```python
from build123d import *

# Parameters (mm, degrees)
BASPROSKE_W             = 5
BASPROSKE_H             = 10.125
TOOTHCUT_DEPTH          = 16.166781135
TEETHCUTS_COUNT         = 13
TEETHCUTS_ANGLE         = 270
BORSKE_R                = 2.5
BORE_DEPTH              = 50.0000508
ENL_V_START             = -10
ENL_V_MAT_EXTRU_1_DEPTH = 10
ESQUISSE2_R             = 1.5
BOSS_EXTRU_1_DEPTH      = 5
BOSS_EXTRU_2_START      = -1
ESQUISSE3_R             = 2.5
BOSS_EXTRU_2_DEPTH      = 4
ESQUISSE4_R             = 1
ENL_V_MAT_EXTRU_2_DEPTH = 10
CONG_1_R                = 5
CONG_2_R                = 8
ENL_V_MAT_EXTRU_4_DEPTH = 2.1
ESQUISSE8_R             = 0.515
ENL_V_MAT_EXTRU_5_DEPTH = 33.049570744


with BuildPart() as part:
    # BasProSke → Base-Revolve (revolve)
    with BuildSketch(Plane(origin=(0, 0, 0), x_dir=(1, 0, 0), z_dir=(0, 1, 0)), mode=Mode.PRIVATE) as base_revolve_sk:
        with Locations((2.5, 5.0625)):
            Rectangle(BASPROSKE_W, BASPROSKE_H)
    revolve(base_revolve_sk.sketch.rotate(Axis((-10, 0, 0), (1, 0, 0)), 180), axis=Axis((-10, 0, 0), (1, 0, 0)))

    # TooCutSke → ToothCut (cut, through all)
    with BuildSketch(Plane(origin=(0, 0, 0), x_dir=(0, 0, -1), z_dir=(1, 0, 0))):
        with BuildLine():
            ThreePointArc((0.588166249, 7.56993481), (0, 7.59275), (-0.588166249, 7.56993481))
            ThreePointArc((-0.588166249, 7.56993481), (-0.930156891, 8.896709021), (-1.743114395, 9.999608611))
            ThreePointArc((-1.743114395, 9.999608611), (0, 10.1504), (1.743114395, 9.999608611))
            ThreePointArc((1.743114395, 9.999608611), (0.930156891, 8.896709021), (0.588166249, 7.56993481))
        make_face()
    toothcut = extrude(amount=TOOTHCUT_DEPTH, mode=Mode.SUBTRACT)

    # TeethCuts: ToothCut ×13 about axis
    teethcuts_axis = Axis((-10, 0, 0), (1, 0, 0))
    for i in range(1, TEETHCUTS_COUNT):
        add(toothcut.rotate(teethcuts_axis, i * TEETHCUTS_ANGLE / (TEETHCUTS_COUNT - 1)), mode=Mode.SUBTRACT)

    # BorSke → Bore (cut, symmetric)
    with BuildSketch(Plane(origin=(0, 0, 0), x_dir=(0, 0, -1), z_dir=(1, 0, 0))):
        with Locations(Location((0, 0, 0), (0, 0, 180))):
            Circle(BORSKE_R)
    extrude(amount=BORE_DEPTH, both=True, mode=Mode.SUBTRACT)

    # Esquisse1 → Enlèv. mat.-Extru.1 (cut)
    with BuildSketch(Plane(origin=(5, 0, 0), x_dir=(0, 0, -1), z_dir=(1, 0, 0)).offset(ENL_V_START)):
        with BuildLine():
            ThreePointArc((7.56993481, 0.588166249), (5.368885013, 5.368885013), (0.588166249, 7.56993481))
            ThreePointArc((0.588166249, 7.56993481), (0.923336805, 8.882279141), (1.719727125, 9.977883724))
            ThreePointArc((1.719727125, 9.977883724), (7.15945616, 7.15945616), (9.977883724, 1.719727125))
            ThreePointArc((9.977883724, 1.719727125), (8.882279141, 0.923336805), (7.56993481, 0.588166249))
        make_face()
    extrude(amount=ENL_V_MAT_EXTRU_1_DEPTH, mode=Mode.SUBTRACT)

    # Esquisse2 → Boss.-Extru.1 (add, through all)
    with BuildSketch(Plane(origin=(5, 0, 0), x_dir=(0, 0, -1), z_dir=(1, 0, 0))):
        with BuildLine():
            Line((16.142135624, 21.46674159), (2, 7.324605966))
            ThreePointArc((2, 7.324605966), (5.368885013, 5.368885013), (7.324605966, 2))
            Line((7.324605966, 2), (21.46674159, 16.142135624))
            ThreePointArc((21.46674159, 16.142135624), (21.46674159, 21.46674159), (16.142135624, 21.46674159))
        make_face()
        with Locations((18.804438607, 18.804438607)):
            Circle(ESQUISSE2_R, mode=Mode.SUBTRACT)
    extrude(amount=-BOSS_EXTRU_1_DEPTH)

    # Esquisse3 → Boss.-Extru.2 (add, through all)
    with BuildSketch(Plane(origin=(5, 0, 0), x_dir=(0, 0, -1), z_dir=(1, 0, 0)).offset(BOSS_EXTRU_2_START)):
        with Locations(Location((0, 0, 0), (0, 0, 180))):
            Circle(ESQUISSE3_R)
    extrude(amount=-BOSS_EXTRU_2_DEPTH)

    # Esquisse4 → Enlèv. mat.-Extru.2 (cut)
    with BuildSketch(Plane(origin=(4, 0, 0), x_dir=(0, 0, -1), z_dir=(1, 0, 0))):
        Circle(ESQUISSE4_R)
    extrude(amount=-ENL_V_MAT_EXTRU_2_DEPTH, mode=Mode.SUBTRACT)

    # Congé1
    cong_1_edges = [part.edges().sort_by_distance(p)[0] for p in [
        (2.5, 7.324605966, -2),
    ]]
    fillet(cong_1_edges, radius=CONG_1_R)

    # Congé2
    cong_2_edges = [part.edges().sort_by_distance(p)[0] for p in [
        (2.5, 2, -7.324605966),
    ]]
    fillet(cong_2_edges, radius=CONG_2_R)

    # Esquisse6 → Enlèv. mat.-Extru.4 (cut)
    with BuildSketch(Plane(origin=(5, 0, 0), x_dir=(0, 0, -1), z_dir=(1, 0, 0))):
        with BuildLine():
            Line((-0.486746212, 3.465988766), (1.140136775, 5.092871753))
            ThreePointArc((1.140136775, 5.092871753), (4.507727263, 5.08472958), (4.91940393, 1.742386942))
            Line((4.91940393, 1.742386942), (3.499344691, -0.067725445))
            ThreePointArc((3.499344691, -0.067725445), (2.619022446, -2.321792719), (0.486746212, -3.465988766))
            Line((0.486746212, -3.465988766), (-1.140072016, -5.092806994))
            ThreePointArc((-1.140072016, -5.092806994), (-4.507662796, -5.08478673), (-4.919460458, -1.742458998))
            Line((-4.919460458, -1.742458998), (-3.499344691, 0.067725445))
            ThreePointArc((-3.499344691, 0.067725445), (-2.619022446, 2.321792719), (-0.486746212, 3.465988766))
        make_face()
    extrude(amount=-ENL_V_MAT_EXTRU_4_DEPTH, mode=Mode.SUBTRACT)

    # Esquisse8 → Enlèv. mat.-Extru.5 (cut, through all)
    with BuildSketch(Plane(origin=(2.9, 0, 0), x_dir=(0, 0, -1), z_dir=(1, 0, 0))):
        with Locations((-2.81931973, -3.180241541)):
            Circle(ESQUISSE8_R)
        with Locations((2.81931973, 3.180241541)):
            Circle(ESQUISSE8_R)
    extrude(amount=-ENL_V_MAT_EXTRU_5_DEPTH, mode=Mode.SUBTRACT)


solid = part.part
```
Model file for the job. Use its own axes, mm. A direction names the side the tool comes from. Coordinates: 2 decimals unless noted, no trailing zeros. Write each loop counter-clockwise with the first axis right and the second up, starting at its lowest first coordinate (ties: lowest second). Pieces come first, ordered by that corner, then holes. Notation, with made-up numbers: (76, -25) - (130, -25) arc R16 cw to (130, -7) - close; hole circle Ø8 at (1.5, 28). An arc over 180 degrees is marked (long way). One line per question, with ' | ' between items. Start each with the question number.
Q1. Cut at B-B, the plane x = 4. Give the number of separate pieces and of enclosed holes in the cut face, then the cut area to 3 significant figures.
Q2. Pull direction Z, two halves, no side cores. Call faces 4 (the face through (3.96, 0.85, -4.22)), 5 (the face through (2.54, 21.41, -21.52)), 6 (the face through (5, 6, -6)): pulls with the +Z half, pulls with the -Z half, needs draft (parallel to the pull), parting line crosses it, or undercut.
Q3. 3-axis set-ups, long thin cutter, end or side, ignore diameter. For faces 1 (the face through (3.96, -0.85, 4.22)), 2 (the face through (2.46, -7.87, 4.27)), 3 (the face through (2.465, 5.375, 5.363)): which of +Z, -Z, +X, -X, +Y, -Y reach the whole face in a straight line?
Q4. Pin check, flat tips, straight feed: pin 1 (1.6 mm diameter, centred on y = -3.18, z = 2.82, fed in from +X); pin 2 (1 mm diameter, centred on x = 1, y = 17, fed in from +Z); pin 3 (3.5 mm diameter, centred on y = 18.8, z = -18.8, fed in from +X); pin 4 (3 mm diameter, centred on x = 4, y = -6.5, fed in from +Z). Stop position of each tip, or through.
Q5. Cut at A-A, the plane y = 11.5. List the corners of the cut face in (x, z).
Q6. Drill centre lines: line 1 (Z direction, x = 3.85, y = -8); line 2 (Z direction, x = 3.15, y = 8.5); line 3 (Z direction, x = 4.35, y = -5.5). Where is each one in solid material? Low to high. Write a range as [from, to].
Answer below:
1) separate pieces: 1 | enclosed holes: 2 | area: 320 mm^2
2) face 4: undercut | face 5: parting line crosses it | face 6: needs draft
3) face 1: +X | face 2: +X, -X, -Y | face 3: +X, -X
4) pin 1: x = 2.9 | pin 2: z = -11.18 | pin 3: x = 5 | pin 4: z = 8.56
5) outline: (0, -16.82) - (5, -16.82) - (5, -6.18) - (0, -6.18) - close
6) line 1: [-5.84, -4.42], [-2.53, -0.64], [0.64, 2.53], [4.42, 5.84] | line 2: [-13.82, -3.07], [0.77, 2.55], [5.26, 5.5] | line 3: [-8.5, -6.62], [-5.23, 1.77], [3.87, 5.23], [6.62, 8.5]
